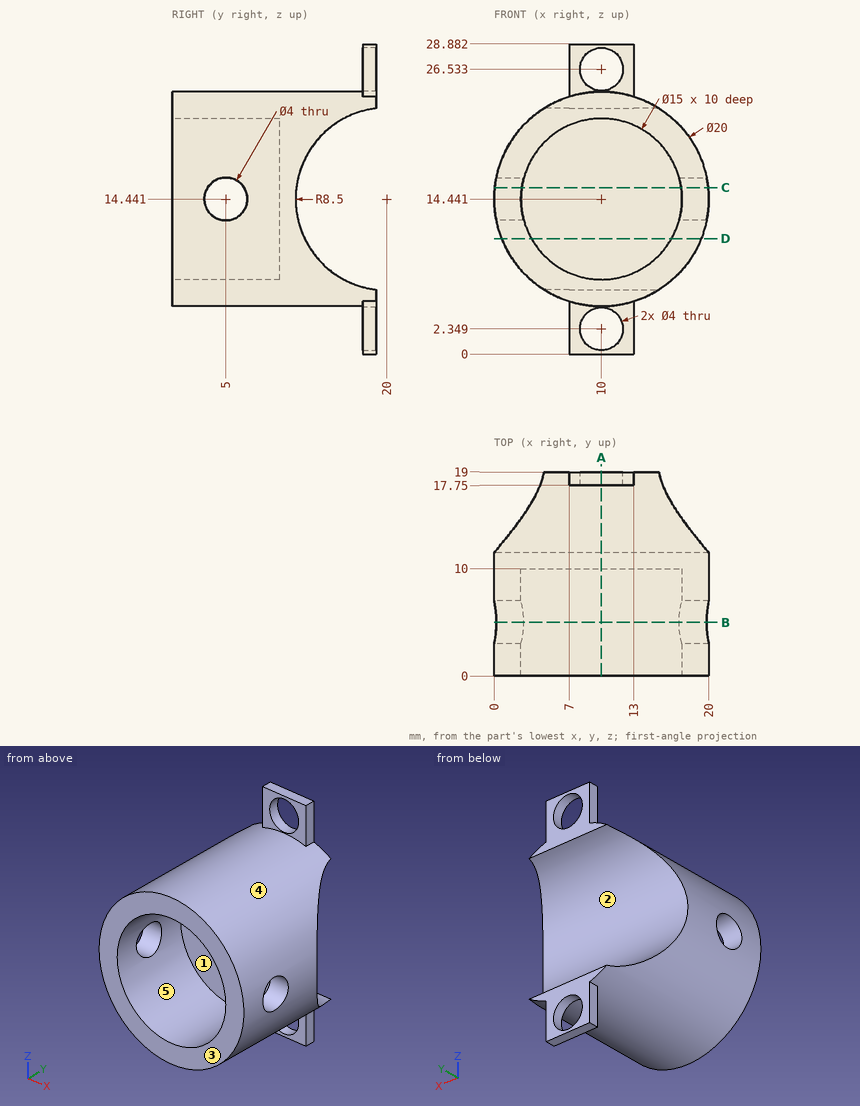
Geometry: see drawing. Coordinates: mm, zero at the bounding-box minimum. A direction names the side the tool comes from. Give positions to 0.01 mm unless a question says otherwise; leave off trailing zeros. Write each loop counter-clockwise with the first axis right and the second up, starting at its lowest first coordinate (ties: lowest second). Pieces come first, ordered by that corner, then holes. Notation, with made-up numbers: M 71,-11.5 L 93,-11.5 A12 cw 93,0.5 Z; hole C 43,30 d5. An arc over 180 degrees is marked long. Answer in a Markdown table with one row per item. Add a question column.
(1) Section A-A on x = 10. Return loops of the section in (y, z), and give its area (3 significant figures).
(2) Section B-B on y = 5. Return loops of the section in (x, z), and give its area (3 significant figures).
(3) Ray query, line 1 (Z direction, x = 10, y = 2); line 2 (Y direction, x = 11.5, z = 4); line 3 (Z direction, x = 4, y = 4.75). Return the intervals inside material, ascending.
(4) Section D-D on z = 10.75. Return loops of the section in (x, y).
(5) Reachability of the marked faces 1 and 2 from +Z, -Z, +X, -X, +Y, -Y: full face, straight path, thin tool, end or side. Return the list, or none.
(6) First-contact query: pin 1 (1.5 mm diameter, centred on y = 17, z = 23, fed in from -X); pin 2 (1 mm diameter, centred on y = 18, z = 27.5, fed in from +X); pin 3 (5 mm diameter, centred on x = 4.5, y = 12, fed in from +Z); pin 4 (3 mm diameter, centred on y = 5, z = 14.44, fed in from -X). Flat tips, straight axial feed; report the tip coordinate or a pass-through.
(7) Section C-C on z = 15.5. Return loops of the section in (x, y) (1 decimal).
(8) Mould query, pull axis X, two halves, no side actions, for the marked faces 3, 4 and 5. Classes: +X half, -X half, draft (parallel to the pull), parting line (faces both ways), or undercut.
Result set:
| question | item | result |
|---|---|---|
| 1 | outline | M 0,4.44 L 17.75,4.44 L 17.75,4.35 L 19,4.35 L 19,6 A8.5 cw 19,22.88 L 19,24.53 L 17.75,24.53 L 17.75,24.44 L 0,24.44 L 0,21.94 L 10,21.94 L 10,6.94 L 0,6.94 Z; M 17.75,0 L 19,0 L 19,0.35 L 17.75,0.35 Z; M 17.75,28.53 L 19,28.53 L 19,28.88 L 17.75,28.88 Z |
| 1 | area | 135 mm^2 |
| 2 | outline | M 0.2,12.44 A10 ccw 19.8,12.44 L 17.23,12.44 A7.5 cw 2.77,12.44 Z; M 0.2,16.44 L 2.77,16.44 A7.5 cw 17.23,16.44 L 19.8,16.44 A10 ccw Z |
| 2 | area | 117 mm^2 |
| 3 | line 1 | z = 4.44 to 6.94, 21.94 to 24.44 |
| 3 | line 2 | y = 17.75 to 19 |
| 3 | line 3 | z = 6.44 to 9.94, 18.94 to 22.44 |
| 4 | outline | M 0.71,0 L 3.47,0 L 3.47,10 L 16.53,10 L 16.53,0 L 19.29,0 L 19.29,12.34 L 0.71,12.34 Z |
| 5 | face 1 | -Y |
| 5 | face 2 | +X, -X, +Y |
| 6 | pin 1 | stops at x = 3.81 |
| 6 | pin 2 | stops at x = 13 |
| 6 | pin 3 | stops at z = 23.98 |
| 6 | pin 4 | passes through |
| 7 | outline | M 0.1,0 L 2.6,0 L 2.6,3.3 L 0.1,3.3 Z; M 0.1,6.7 L 2.6,6.7 L 2.6,10 L 17.4,10 L 17.4,6.7 L 19.9,6.7 L 19.9,11.6 L 0.1,11.6 Z; M 17.4,0 L 19.9,0 L 19.9,3.3 L 17.4,3.3 Z |
| 8 | face 3 | draft |
| 8 | face 4 | parting line |
| 8 | face 5 | undercut |
